Geometry: see drawing. Coordinates: mm, zero at the bounding-box minimum. Coordinates: 2 decimals unless noted, no trailing zeros. Write each loop counter-clockwise with the first axis right and the second up, starting at its lowest first coordinate (ties: lowest second). Pieces come first, ordered by that corner, then holes.
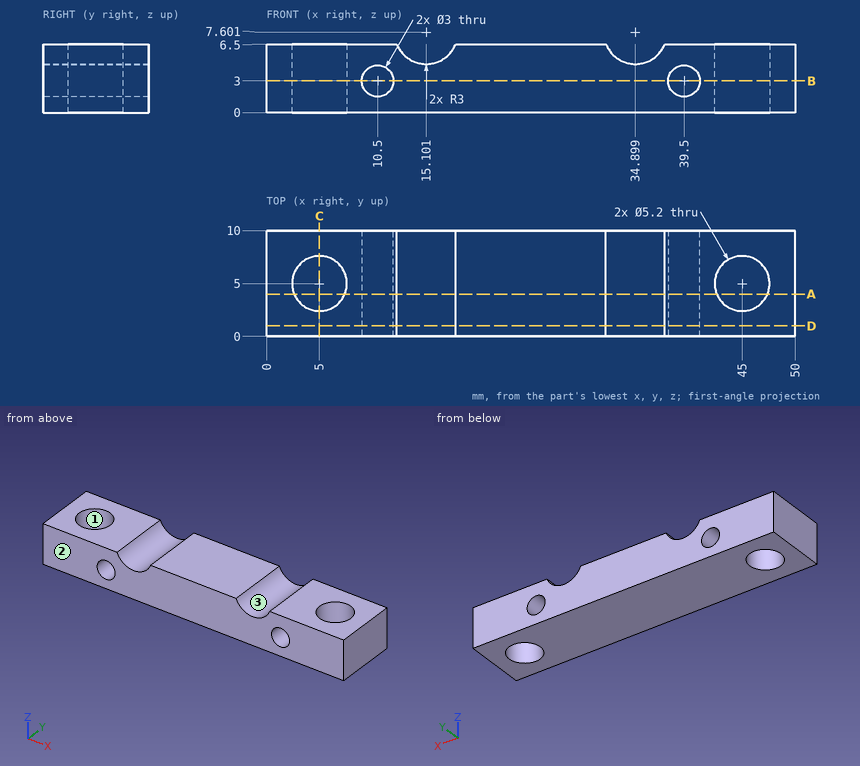
Item 1: Section A-A, the plane y = 4. Output: boundary loops of the cut face in (x, z), plus the area to 3 significant figures.
Derived:
outline: (0, 0) - (2.6, 0) - (2.6, 6.5) - (0, 6.5) - close; (7.4, 0) - (42.6, 0) - (42.6, 6.5) - (37.69, 6.5) arc R3 cw to (32.11, 6.5) - (17.89, 6.5) arc R3 cw to (12.31, 6.5) - (7.4, 6.5) - close; (47.4, 0) - (50, 0) - (50, 6.5) - (47.4, 6.5) - close; hole circle Ø3 at (10.5, 3); hole circle Ø3 at (39.5, 3)
area: 233 mm2
Item 2: Section C-C, the plane x = 5. Output: boundary loops of the cut face in (y, z).
Derived:
outline: (0, 0) - (2.4, 0) - (2.4, 6.5) - (0, 6.5) - close; (7.6, 0) - (10, 0) - (10, 6.5) - (7.6, 6.5) - close
Item 3: Pull-direction query (Y, two-part tool) for the marked faces 1, 2 and 3; classes: released by +Y, released by -Y, zero draft, split by the parting line, or undercut.
Derived:
face 1: undercut
face 2: released by -Y
face 3: zero draft
Item 4: Section B-B, the plane z = 3. Output: boundary loops of the cut face in (x, y).
Derived:
outline: (0, 0) - (9, 0) - (9, 10) - (0, 10) - close; (12, 0) - (38, 0) - (38, 10) - (12, 10) - close; (41, 0) - (50, 0) - (50, 10) - (41, 10) - close; hole circle Ø5.2 at (5, 5); hole circle Ø5.2 at (45, 5)
Item 5: Material intervals for probe 1 along X at (y, z) = (5.25, 3); probe 2 along Z at (x, y) = (10.5, 7.25); probe 3 along X at (y, z) = (1.5, 5.75), sorted ascending.
Derived:
probe 1: x = 0 to 2.41, 7.59 to 9, 12 to 38, 41 to 42.41, 47.59 to 50
probe 2: z = 0 to 1.5, 4.5 to 6.5
probe 3: x = 0 to 12.74, 17.46 to 32.54, 37.26 to 50
Item 6: Section D-D, the plane y = 1. Output: boundary loops of the cut face in (x, z).
Derived:
outline: (0, 0) - (50, 0) - (50, 6.5) - (37.69, 6.5) arc R3 cw to (32.11, 6.5) - (17.89, 6.5) arc R3 cw to (12.31, 6.5) - (0, 6.5) - close; hole circle Ø3 at (10.5, 3); hole circle Ø3 at (39.5, 3)
Item 7: Pin query (flat end, axial travel): pin 1 (4 mm diameter, centred on x = 5, y = 5, fed in from +Z); pin 2 (4 mm diameter, centred on x = 10.5, y = 6.5, fed in from -Z). Return the tip coordinate at first contact, or that it passes through.
Derived:
pin 1: passes through
pin 2: stops at z = 0
